CAD build for the part. Positions are in the model's coordinates, mm. A direction names the side the tool comes from. Round coordinates to 2 decimals unless told otherwise and drop trailing zeros. Loops run counter-clockwise (first coordinate to the right, second up) from the corner with the lowest first, then second, coordinate; pieces in that order, holes last. Notation, with made-up numbers: (37.5, 34) -> (92.5, 34) arc R30 ccw to (92.5, 66) -> close; hole circle Ø9 at (-13.5, 59). An arc over 180 degrees is marked (long way). Answer as CSV lines item,"result".
```python
from build123d import *
from OCP.BRepFilletAPI import BRepFilletAPI_MakeChamfer

# Parameters (mm, degrees)
SKETCH1_W           = 1243.0125
SKETCH1_H           = 304.8
BOSS_EXTRUDE1_DEPTH = 19.05
CUT_EXTRUDE2_DEPTH  = 641.202062859
SKETCH5_W           = 114.3
SKETCH5_H           = 152.4
CUT_EXTRUDE3_DEPTH  = 641.202062859
SKETCH6_R           = 12.7
CUT_EXTRUDE4_DEPTH  = 641.202062859
CHAMFER1_SIZE       = 19.05
CHAMFER1_SIZE_2     = 4.0492025
SKETCH8_R           = 1.65
CUT_EXTRUDE5_DEPTH  = 641.202062859


with BuildPart() as part:
    # Sketch1 → Boss-Extrude1 (new body)
    with BuildSketch(Plane(origin=(0, 0, 0), x_dir=(1, 0, 0), z_dir=(0, 1, 0))):
        Rectangle(SKETCH1_W, SKETCH1_H)
    extrude(amount=BOSS_EXTRUDE1_DEPTH)

    # Sketch4 → Cut-Extrude2 (cut, through all)
    with BuildSketch(Plane(origin=(0, 19.05, 0), x_dir=(1, 0, 0), z_dir=(0, 1, 0))):
        with BuildLine():
            Line((-418.30625, -152.4), (-418.30625, -63.5))
            ThreePointArc((-418.30625, -63.5), (-399.707530605, -18.598719395), (-354.80625, 0))
            Line((-354.80625, 0), (-253.20625, 0))
            ThreePointArc((-253.20625, 0), (-208.304969395, -18.598719395), (-189.70625, -63.5))
            Line((-189.70625, -63.5), (-189.70625, -152.4))
            Line((-189.70625, -152.4), (-418.30625, -152.4))
        make_face()
        with BuildLine():
            Line((189.70625, -152.4), (189.70625, -63.5))
            ThreePointArc((189.70625, -63.5), (208.304969395, -18.598719395), (253.20625, 0))
            Line((253.20625, 0), (354.80625, 0))
            ThreePointArc((354.80625, 0), (399.707530605, -18.598719395), (418.30625, -63.5))
            Line((418.30625, -63.5), (418.30625, -152.4))
            Line((418.30625, -152.4), (189.70625, -152.4))
        make_face()
    extrude(amount=-CUT_EXTRUDE2_DEPTH, mode=Mode.SUBTRACT)

    # Sketch5 → Cut-Extrude3 (cut, through all)
    with BuildSketch(Plane(origin=(0, 19.05, 0), x_dir=(1, 0, 0), z_dir=(0, 1, 0))):
        with Locations((0, -50.8)):
            Rectangle(SKETCH5_W, SKETCH5_H)
    extrude(amount=-CUT_EXTRUDE3_DEPTH, mode=Mode.SUBTRACT)

    # Sketch6 → Cut-Extrude4 (cut, through all)
    with BuildSketch(Plane(origin=(0, 19.05, 0), x_dir=(1, 0, 0), z_dir=(0, 1, 0))):
        with Locations(Location((-532.60625, -101.6, 0), (0, 0, 270))):
            Circle(SKETCH6_R)
        with Locations(Location((532.60625, -101.6, 0), (0, 0, 270))):
            Circle(SKETCH6_R)
    extrude(amount=-CUT_EXTRUDE4_DEPTH, mode=Mode.SUBTRACT)

    # Chamfer1
    chamfer1_edges_1 = [part.edges().sort_by_distance(p)[0] for p in [
        (519.90625, 19.05, 152.4),
    ]]
    chamfer1_side_1 = [part.faces().sort_by_distance(p)[0] for p in [
        (519.90625, 18.96901595, 152.4),
    ]]
    chamfer1_edges_2 = [part.edges().sort_by_distance(p)[0] for p in [
        (0, 19.05, 152.4),
    ]]
    chamfer1_side_2 = [part.faces().sort_by_distance(p)[0] for p in [
        (0, 19.05, 152.31901595),
    ]]
    chamfer1_edges_3 = [part.edges().sort_by_distance(p)[0] for p in [
        (-519.90625, 19.05, 152.4),
    ]]
    chamfer1_side_3 = [part.faces().sort_by_distance(p)[0] for p in [
        (-519.90625, 19.05, 152.31901595),
    ]]
    chamfer1 = BRepFilletAPI_MakeChamfer(part.part.solid().wrapped)
    for e in chamfer1_edges_1:
        chamfer1.Add(CHAMFER1_SIZE - 0.0001, CHAMFER1_SIZE_2 - 0.0001, e.wrapped, chamfer1_side_1[0].wrapped)
    for e in chamfer1_edges_2:
        chamfer1.Add(CHAMFER1_SIZE_2 - 0.0001, CHAMFER1_SIZE - 0.0001, e.wrapped, chamfer1_side_2[0].wrapped)
    for e in chamfer1_edges_3:
        chamfer1.Add(CHAMFER1_SIZE_2 - 0.0001, CHAMFER1_SIZE - 0.0001, e.wrapped, chamfer1_side_3[0].wrapped)
    add(Compound.cast(chamfer1.Shape()), mode=Mode.REPLACE)  # a hair under: the kernel refuses the full size

    # Sketch8 → Cut-Extrude5 (cut, through all)
    with BuildSketch(Plane(origin=(0, 19.05, 0), x_dir=(1, 0, 0), z_dir=(0, 1, 0))):
        with Locations(Location((-564.50625, -25.4, 0), (0, 0, 270))):
            Circle(SKETCH8_R)
        with Locations(Location((-564.50625, -49.7, 0), (0, 0, 270))):
            Circle(SKETCH8_R)
        with Locations(Location((-500.70625, -49.7, 0), (0, 0, 270))):
            Circle(SKETCH8_R)
        with Locations(Location((-500.70625, -25.4, 0), (0, 0, 270))):
            Circle(SKETCH8_R)
        with Locations(Location((500.70625, -25.4, 0), (0, 0, 270))):
            Circle(SKETCH8_R)
        with Locations(Location((500.70625, -49.7, 0), (0, 0, 270))):
            Circle(SKETCH8_R)
        with Locations(Location((564.50625, -49.7, 0), (0, 0, 270))):
            Circle(SKETCH8_R)
        with Locations(Location((564.50625, -25.4, 0), (0, 0, 270))):
            Circle(SKETCH8_R)
        with BuildLine():
            Line((-513.40625, -51.05), (-551.80625, -51.05))
            ThreePointArc((-551.80625, -51.05), (-565.30625, -37.55), (-551.80625, -24.05))
            Line((-551.80625, -24.05), (-513.40625, -24.05))
            ThreePointArc((-513.40625, -24.05), (-499.90625, -37.55), (-513.40625, -51.05))
        make_face()
        with BuildLine():
            Line((513.40625, -51.05), (551.80625, -51.05))
            ThreePointArc((551.80625, -51.05), (565.30625, -37.55), (551.80625, -24.05))
            Line((551.80625, -24.05), (513.40625, -24.05))
            ThreePointArc((513.40625, -24.05), (499.90625, -37.55), (513.40625, -51.05))
        make_face()
    extrude(amount=-CUT_EXTRUDE5_DEPTH, mode=Mode.SUBTRACT)


solid = part.part
```
Q1. Probe L1, parallel to X at y = 8, z = 101.6; L2, parallel to X at y = 18, z = 81; L3, parallel to Z at x = -542, y = 17. List the from-to ranges inside material, lowest first. Write a range as [from, to].
Results:
L1,"[-621.51, -545.31], [-519.91, -418.31], [-189.71, -57.15], [57.15, 189.71], [418.31, 519.91], [545.31, 621.51]"
L2,"[-621.51, -418.31], [-189.71, -57.15], [57.15, 189.71], [418.31, 621.51]"
L3,"[-152.4, 24.05], [51.05, 93.05], [110.15, 148.79]"
Q2. Slice it at D-D, the plane y = 15.5. Count the separate pieces of the cut face and the enclosed holes in it, and give its area (3 significant figures).
Results:
separate pieces,"1"
enclosed holes,"13"
area,"288,000 mm2"
Q3. Two-plate mould, pull along X, no slides. Class faces 3 (the flat face through (-9, 0, -36)), 4 (the cylindrical face through (-528.792, 9.658, 113.714)): pulls with the +X half, pulls with the -X half, needs draft (parallel to the pull), parting line crosses it, or undercut.
Results:
face 3,"needs draft"
face 4,"undercut"
Q4. Slice it at A-A, the plane z = 101.6. Give the cut face in (x, y).
Results:
outline,"(-621.51, 0) -> (-545.31, 0) -> (-545.31, 19.05) -> (-621.51, 19.05) -> close; (-519.91, 0) -> (-418.31, 0) -> (-418.31, 19.05) -> (-519.91, 19.05) -> close; (-189.71, 0) -> (-57.15, 0) -> (-57.15, 19.05) -> (-189.71, 19.05) -> close; (57.15, 0) -> (189.71, 0) -> (189.71, 19.05) -> (57.15, 19.05) -> close; (418.31, 0) -> (519.91, 0) -> (519.91, 19.05) -> (418.31, 19.05) -> close; (545.31, 0) -> (621.51, 0) -> (621.51, 19.05) -> (545.31, 19.05) -> close"
Q5. Drop flat-ended pins along their axis: pin 1 Ø5.5 at (x, y) = (-541.5, 9) entering from +Z; pin 2 Ø1 at (x, y) = (-369.5, 9.5) entering from +Z; pin 3 Ø5.5 at (x, y) = (532, 12.5) entering from +Z. Give the stop position or say it passes through.
Results:
pin 1,"z = 151.07"
pin 2,"z = 1.84"
pin 3,"z = 150.33"
Q6. Slice it at C-C, the plane x = 330. Give the cut face in (y, z), and give its area (3 significant figures).
Results:
outline,"(0, -152.4) -> (19.05, -152.4) -> (19.05, 0) -> (0, 0) -> close"
area,"2,900 mm2"
Q7. Tool access for faces 1 (the cylindrical face through (399.211, 9.658, 18.108)), 2 (the cylindrical face through (545.2, 9.66, 99.95)): list every direction of +Z, -Z, +X, -X, +Y, -Y with a clear straight run to the whole face (end or side of a thin tool).
Results:
face 1,"+Z, +Y, -Y"
face 2,"+Y, -Y"
Q8. Slice it at B-B, the plane z = 37.55. Give the cut face in (x, y).
Results:
outline,"(-621.51, 0) -> (-565.31, 0) -> (-565.31, 19.05) -> (-621.51, 19.05) -> close; (-499.91, 0) -> (-412.76, 0) -> (-412.76, 19.05) -> (-499.91, 19.05) -> close; (-195.25, 0) -> (-57.15, 0) -> (-57.15, 19.05) -> (-195.25, 19.05) -> close; (57.15, 0) -> (195.25, 0) -> (195.25, 19.05) -> (57.15, 19.05) -> close; (412.76, 0) -> (499.91, 0) -> (499.91, 19.05) -> (412.76, 19.05) -> close; (565.31, 0) -> (621.51, 0) -> (621.51, 19.05) -> (565.31, 19.05) -> close"
